Here's how the part is built. I have some questions about the finished solid (model axes, mm). A direction names the side the tool comes from. Round coordinates to 2 decimals unless told otherwise and drop trailing zeros. Loops run counter-clockwise (first coordinate to the right, second up) from the corner with the lowest first, then second, coordinate; pieces in that order, holes last. Notation, with made-up numbers: M 68,51.5 L 126,51.5 A7 cw 126,61.5 Z; hole C -22,6 d6. An arc over 180 degrees is marked long. Write each question's results on one line, items separated by ' | '. Start each with the question number.
```python
from build123d import *

# Parameters (mm, degrees)
F2_SIZE  = 0.5
F3_SIZE  = 0.75
F4_R     = 5
F5_DEPTH = 10.501


with BuildPart() as f1:
    # F0 (on Front) → F1 (revolve)
    with BuildSketch(Plane.XZ):
        Polygon((0.2, 1.5), (0.2, 0), (0.6, 0), (2.1, 2), (4.2, 2), (4.2, 5), (2.4, 5), (2.4, 6.5), (3, 6.5), (3, 12.5), (1, 12.5), (1, 1.980688), align=None)
    revolve(axis=Axis((0, 0, 6.25), (0, 0, 1)))

    # F2
    f2_edges = [f1.edges().sort_by_distance(p)[0] for p in [
        (-3, 0, 6.5),
        (-3, 0, 12.5),
    ]]
    chamfer(f2_edges, length=F2_SIZE)

    # F3
    f3_edges = [f1.edges().sort_by_distance(p)[0] for p in [
        (-1, 0, 12.5),
    ]]
    chamfer(f3_edges, length=F3_SIZE)

    # F4 (on face) → F5 (cut, through all)
    with BuildSketch(Plane(origin=(0, 0, 2), x_dir=(1, 0, 0), z_dir=(0, 0, -1))):
        Circle(F4_R)
        Polygon((2.020726, -3.5), (-2.020726, -3.5), (-4.041452, 0), (-2.020726, 3.5), (2.020726, 3.5), (4.041452, 0), align=None, mode=Mode.SUBTRACT)
    extrude(amount=-F5_DEPTH, mode=Mode.SUBTRACT)


solid = f1.part
```
Item 1: I'm going to push flat-ended pins straight in: pin 1 (2 mm diameter, centred on x = 1.5, y = 1, fed in from -Z); pin 2 (1 mm diameter, centred on y = 1, z = 2, fed in from +X). Where does each tip first touch, or does it pass through?
Item 2: If we section it at B-B on z = 6.75: Please give me the cut outline in (x, y), and give its area (3 significant figures).
Item 3: If we mould it in two halves opening along X, with no side actions, what happens to faces 4 (the face through (-3, 0, 10)), 5 (the face through (3, 0, 5)), 6 (the face through (0, -1, 7))? For each: released by +X, released by -X, zero draft, split by the parting line, or undercut.
Item 4: Which directions (+Z, -Z, +X, -X, +Y, -Y) give clear straight access to the entire face, cutting with the end or side of a thin tool? Please do faces 1 (the face through (-3, 1.8, 3.5)), 2 (the face through (-2, 2, 2)), 3 (the face through (1.29, 2.024, 5.76)).
Item 5: I need wall thicknesses on L1, parallel to Z at x = -1.75, y = 1.75; L2, parallel to Z at x = -2.75, y = -0.5; L3, parallel to Z at x = -3.25, y = -1. Which ranges of each line are inside material? Lowest first, please.
Numbers:
1) pin 1: z = 0.27 | pin 2: x = 3.75
2) outline: C 0,0 d5.5; hole C 0,0 d2 | area: 20.6 mm²
3) face 4: split by the parting line | face 5: zero draft | face 6: undercut
4) face 1: +Z, -Z, -X, +Y | face 2: -Z | face 3: none
5) L1: 2 to 5, 6.5 to 12.5 | L2: 2 to 5, 6.8 to 12.2 | L3: 2 to 5
